CAD build for the part. Positions are in the model's coordinates, mm. A direction names the side the tool comes from. Round coordinates to 2 decimals unless told otherwise and drop trailing zeros. Order: outer loops, then holes, each group sorted by start corner. A loop starts at its lowest first (then second) coordinate and runs counter-clockwise, first axis right, second up. Notation, with made-up numbers: (52, -5) -> (59, -5) arc R23 ccw to (59, 21) -> close; hole circle Ø6 at (-30.75, 38). An arc over 180 degrees is marked (long way). Return JSON: item names as keys, results as strings. Group by question number.
Q1. Flat gauge pins, fed straight in: pin 1 (3 mm diameter, centred on x = 3.39, y = -3.3, fed in from -Z); pin 2 (9 mm diameter, centred on x = 28.5, y = -17, fed in from +Z); pin 3 (6 mm diameter, centred on y = -20, z = -15.5, fed in from +X); pin 4 (2 mm diameter, centred on x = 25.5, z = -6, fed in from +Y). Where does each tip first touch, or does it go through?
Q2. Cut at C-C (z = -7). Write the cut outline in (x, y) (3 decimals).
Q3. Probe line 1 along Y through (x, z) = (32.35, 3.3); line 2 along Y through (x, z) = (3.39, 2.4); line 3 along X through (y, z) = (-34.5, -0.75) (3 decimals). List the from-to ranges inside material, lowest first.
Q4. Cut at B-B (y = -3.3). Write the cut outline in (x, z).
Q5. Mould opens along X. For faces 1 (the flat face through (5, -12, -6)), 2 (the cylindrical face through (33.185, -12.1, -16.315)), 3 (the flat face through (31.67, -34, 2)) say: +X half, -X half, draft (parallel to the pull), parting line (faces both ways), or undercut.
Q6. Cut at D-D (y = -22). Write the cut outline in (x, z).
Q7. Which spindle directions (+Z, -Z, +X, -X, +Y, -Y) get a long thin tool onto all of the face, cutting with end or side? Do faces 4 (the flat face through (30, -11, 4)), 5 (the flat face through (34, -24, 2)), 6 (the flat face through (35.65, -44.5, 2.5)), 7 (the flat face through (19.825, -38, -8)). Say none if no direction does.
Q8. Cut at A-A (x = 32.35). Write the cut outline in (y, z), then the cut area to 3 significant figures.
Autodesk Inventor part; units mm, degrees
ref_plane "YZ Plane" through (0, 0, 0) normal (1, 0, 0) x (0, 1, 0)
ref_plane "XZ Plane" through (0, 0, 0) normal (0, 1, 0) x (-1, 0, 0)
ref_plane "XY Plane" through (0, 0, 0) normal (0, 0, 1) x (1, 0, 0)
sketch "Эскиз1" plane through (0, 0, 0) normal (0, 0, 1) x (1, 0, 0)
  line L0 (0, 0) -> (35.65, 0)
  line L1 (35.65, 0) -> (35.65, -45)
  line L2 (35.65, -45) -> (0, -45)
  line L3 (0, -45) -> (0, 0)
  dimension "d0" = 35.65
  dimension "d1" = 45
extrude "Выдавливание1" add sketch "Эскиз1" along normal blind 5
sketch "Эскиз5" plane through (0, -45, 0) normal (-1, 0, 0) x (0, 0, 1)
  line L0 (0, 0) -> (0, 45)
  line L1 (0, 26.3892) -> (-12, 28.047)
  circle A0 centre (-11.3157, 33) radius 5
  circle A1 centre (-11.3157, 33) radius 2.1
  line L2 (0, 45) -> (5, 45)
  line L3 (-12, 37.953) -> (0, 40.0416)
  point P0 (0, 38.3892)
  point P1 (-10.5919, 37.9473)
  point P2 (-11.2301, 37.9993)
  point P3 (0, 41.0557)
  dimension "d4" = 4.2
  dimension "d5" = 10
  dimension "d8" = 12
  dimension "d9" = 12
  dimension "d10" = 12
  dimension "d18" = 12
extrude "Выдавливание2" add sketch "Эскиз5" against normal blind 5
ref_plane "РабПлоскость1" through (17.825, -45, 5) normal (-1, 0, 0) x (0, 0, 1)
mirror "Зеркальное отражение1" about plane through (17.825, -45, 5) normal (-1, 0, 0) of "Выдавливание2"
sketch "Эскиз7" plane through (0, 0, 0) normal (0, 0, -1) x (-1, 0, 0)
  circle A0 centre (-32.35, -3.3) radius 1.4
  circle A1 centre (-3.39, -3.3) radius 1.4
  line L0 (-3.9799, -24) -> (1.0201, -24)
  line L1 (1.0201, -24) -> (1.0201, -44)
  line L2 (1.0201, -44) -> (-3.9799, -44)
  line L3 (-3.9799, -44) -> (-3.9799, -24)
  line L4 (0, -45) -> (-35.65, -45) construction
  line L5 (-17.825, -45) -> (-17.825, 0) construction
  line L6 (-35.65, 0) -> (0, 0) construction
  line L7 (-31.6701, -24) -> (-36.6701, -24)
  line L8 (-36.6701, -24) -> (-36.6701, -44)
  line L9 (-36.6701, -44) -> (-31.6701, -44)
  line L10 (-31.6701, -44) -> (-31.6701, -24)
  line L11 (0, 0) -> (0, -45) construction
  point P0 (0, -18.6108)
  dimension "d14" = 1
  dimension "d15" = 20
  dimension "d24" = 5
extrude "Выдавливание3" cut sketch "Эскиз7" against normal through all
sketch "Эскиз9" plane through (0, 0, 5) normal (0, 0, 1) x (1, 0, 0)
  line L0 (35.65, -45) -> (35.65, 0)
  line L1 (35.65, -11) -> (24.65, -11)
  line L2 (24.65, -11) -> (24.65, -23)
  line L3 (24.65, -23) -> (35.65, -23)
  line L4 (35.65, -23) -> (35.65, -11)
  point P0 (0, 0)
  dimension "d19" = 11
  dimension "d20" = 12
  dimension "d21" = 11
extrude "Выдавливание4" cut sketch "Эскиз9" against normal blind 3
ref_plane "РабПлоскость2" through (15.825, -45, 5) normal (-1, 0, 0) x (0, 0, 1)
sketch "Эскиз10" plane through (15.825, -45, 5) normal (-1, 0, 0) x (0, 0, 1)
  circle A0 centre (-20.0926, 6.8885) radius 5.1
  circle A1 centre (-20.0926, 6.8885) radius 2.1
  line L0 (-20.6814, 1.8226) -> (-5, 0)
  line L1 (-5, 11.6783) -> (-5, 0)
  line L2 (-20.4955, 11.9725) -> (-5, 13.2004)
  line L3 (-5, 1) -> (-5, 21)
  point P0 (-5, 45)
  point P1 (-20.9797, 11.9107)
  point P2 (-22.1404, 2.2176)
  point P3 (-20.6271, 11.9604)
  dimension "d28" = 4.2
  dimension "d29" = 10.2
extrude "Выдавливание5" add sketch "Эскиз10" along normal blind 5
mirror "Зеркальное отражение2" about plane through (17.825, -45, 5) normal (-1, 0, 0) of "Выдавливание5"
ref_plane "РабПлоскость3" through (17.825, 0, 5) normal (1, 0, 0) x (0, 0, -1)
properties part number "Качель камеры"
Solution:
{
 "1": {"pin 1": "stops at z = 0", "pin 2": "stops at z = 5", "pin 3": "passes through", "pin 4": "stops at y = -32.22"},
 "2": {"outline": "(0, -17.644) -> (5, -17.644) -> (5, -6.177) -> (0, -6.177) -> close; (10.825, -44.186) -> (15.825, -44.186) -> (15.825, -32.354) -> (10.825, -32.354) -> close; (19.825, -44.186) -> (24.825, -44.186) -> (24.825, -32.354) -> (19.825, -32.354) -> close; (30.65, -17.644) -> (35.65, -17.644) -> (35.65, -6.177) -> (30.65, -6.177) -> close"},
 "3": {"line 1": "y = -45 to -44, -24 to -23, -11 to -4.7, -1.9 to 0", "line 2": "y = -45 to -44, -24 to -4.7, -1.9 to 0", "line 3": "x = 10.825 to 15.825, 19.825 to 24.825"},
 "4": {"outline": "(0, 0) -> (1.99, 0) -> (1.99, 5) -> (0, 5) -> close; (4.79, 0) -> (30.95, 0) -> (30.95, 5) -> (4.79, 5) -> close; (33.75, 0) -> (35.65, 0) -> (35.65, 5) -> (33.75, 5) -> close"},
 "5": {"face 1": "undercut", "face 2": "draft", "face 3": "+X half"},
 "6": {"outline": "(0, 0) -> (35.65, 0) -> (35.65, 2) -> (24.65, 2) -> (24.65, 5) -> (0, 5) -> close"},
 "7": {"face 4": "+Z, +X", "face 5": "+Z, -Z, +X", "face 6": "+Z, -Z, +X, +Y, -Y", "face 7": "-Z, +Y, -Y"},
 "8": {"outline": "(-45, 0) -> (-44, 0) -> (-44, 5) -> (-45, 5) -> close; (-24, 0) -> (-18.61, 0) -> (-16.95, -12) arc R5 ccw to (-7.05, -12) -> (-4.96, 0) -> (-4.7, 0) -> (-4.7, 5) -> (-11, 5) -> (-11, 2) -> (-23, 2) -> (-23, 5) -> (-24, 5) -> close; (-1.9, 0) -> (0, 0) -> (0, 5) -> (-1.9, 5) -> close; hole circle Ø4.2 at (-12, -11.32)", "area": "235 mm²"}
}
